Autodesk Inventor part; units mm, degrees
ref_plane "YZ Plane" through (0, 0, 0) normal (1, 0, 0) x (0, 1, 0)
ref_plane "XZ Plane" through (0, 0, 0) normal (0, 1, 0) x (-1, 0, 0)
ref_plane "XY Plane" through (0, 0, 0) normal (0, 0, 1) x (1, 0, 0)
sketch "Sketch1" plane through (0, 0, 0) normal (0, 0, 1) x (1, 0, 0)
  line L0 (0, 0) -> (50.8, 0)
  line L1 (50.8, 0) -> (50.8, -25.4)
  line L2 (50.8, -25.4) -> (0, -25.4)
  line L3 (0, -25.4) -> (0, 0)
  line L4 (3.175, -3.175) -> (47.625, -3.175)
  line L5 (47.625, -3.175) -> (47.625, -22.225)
  line L6 (47.625, -22.225) -> (3.175, -22.225)
  line L7 (3.175, -22.225) -> (3.175, -3.175)
  dimension "d0" = 50.8
  dimension "d1" = 25.4
  dimension "d2" = 44.45
  dimension "d3" = 19.05
  dimension "d4" = 3.175
  dimension "d5" = 3.175
extrude "Extrusion1" add sketch "Sketch1" along normal blind 584.2
sketch "Sketch2" plane through (0, 0, 0) normal (0, 1, 0) x (1, 0, 0)
  circle A0 centre (12.7, -12.7) radius 3.175
  line L0 (3.175, 0) -> (47.625, 0)
  line L1 (23.7245, 0) -> (23.7245, -584.2)
  line L2 (47.625, -584.2) -> (3.175, -584.2)
  line L3 (23.7245, 0) -> (607.9245, 0) construction
  line L4 (0, 0) -> (0, -584.2)
  circle A1 centre (34.749, -12.7) radius 3.175
  line L5 (0, -311.15) -> (50.8388, -311.15)
  line L6 (47.625, 0) -> (47.625, -584.2)
  circle A2 centre (12.7, -609.6) radius 3.175
  circle A3 centre (34.749, -609.6) radius 3.175
  dimension "d8" = 6.35
  dimension "d9" = 90
  dimension "d10" = 12.7
  dimension "d11" = 12.7
  dimension "d12" = 311.15
hole "Hole1" at (12.7, 0, 609.6) at (34.749, 0, 609.6) at (12.7, 0, 12.7) at (34.749, 0, 12.7) direction (0, -1, 0) diameter 6.35 depth 25.4 tip angle 118
properties part number "support beam 2"
Read the model definition and answer for the solid it produces. Units are mm, in the model's axes. A direction names the side the tool comes from. Round coordinates to 2 decimals unless told otherwise and drop trailing zeros. Write each loop counter-clockwise with the first axis right and the second up, starting at its lowest first coordinate (ties: lowest second). Pieces come first, ordered by that corner, then holes.
Q1. Straight lines are drawn through the part: line 1 (X direction, y = -2.4, z = 12.7) (3 decimals); line 2 (Y direction, x = 42, z = 345) (3 decimals); line 3 (Z direction, x = 12.7, y = -23.1) (3 decimals). For each, find the intervals that lie inside material, in ascending order.
Values:
line 1: x = 0 to 9.525, 15.875 to 31.574, 37.924 to 50.8
line 2: y = -25.4 to -22.225, -3.175 to 0
line 3: z = 0 to 9.525, 15.875 to 584.2
Q2. Find section B-B on z = 79. Determine the outline of the cut face in (x, y) (3 decimals), and give its area (3 significant figures).
Values:
outline: (0, -25.4) - (50.8, -25.4) - (50.8, 0) - (0, 0) - close; hole (3.175, -22.225) - (47.625, -22.225) - (47.625, -3.175) - (3.175, -3.175) - close
area: 444 mm2
Q3. Find section A-A on y = -14.5. Determine the outline of the cut face in (x, z) (3 decimals), and give its area (3 significant figures).
Values:
outline: (0, 0) - (3.175, 0) - (3.175, 584.2) - (0, 584.2) - close; (47.625, 0) - (50.8, 0) - (50.8, 584.2) - (47.625, 584.2) - close
area: 3,710 mm2
Q4. A tool of negligible diameter and unlimited length cuts with its end or side. For faces 5 (the face through (0, -13, 288)), 6 (the face through (3.175, -13, 288)), from which of +Z, -Z, +X, -X, +Y, -Y can it reach the whole face along a straight path? Write none if from no direction.
Values:
face 5: +Z, -Z, -X, +Y, -Y
face 6: +Z, -Z
Q5. The mould has two halves that part along X. Classify faces 1 (the face through (26, -25.4, 288)), 2 (the face through (50.8, -13, 288)), 3 (the face through (26, -22.225, 288)), 4 (the face through (25, -3.175, 288)): released by +X, released by -X, zero draft, split by the parting line, or undercut.
Values:
face 1: zero draft
face 2: released by +X
face 3: undercut
face 4: undercut
Q6. Find section C-C on x = 24.5. Determine the outline of the cut face in (y, z) (3 decimals).
Values:
outline: (-25.4, 0) - (-22.225, 0) - (-22.225, 584.2) - (-25.4, 584.2) - close; (-3.175, 0) - (0, 0) - (0, 584.2) - (-3.175, 584.2) - close
